Can you work these out from the model? Positions are in its coordinate system, mm. Face numbers are marked on the shaded views. A direction names the side the tool comes from. Give positions to 0.01 mm unless a question says otherwise; leave off trailing zeros. Write each loop counter-clockwise with the first axis right and the second up, starting at its lowest first coordinate (ties: lowest second). Pieces come first, ordered by that corner, then holes.
Autodesk Inventor part; units mm, degrees
ref_plane "Work Plane1" through (0, 190, 0) normal (0, 1, 0) x (-1, 0, 0)
ref_plane "Work Plane3" through (135, 0, 0) normal (1, 0, 0) x (0, 1, 0)
ref_plane "XY Plane" through (0, 0, 0) normal (0, 0, 1) x (1, 0, 0)
sketch "Sketch1" plane through (0, 0, 0) normal (0, 0, 1) x (1, 0, 0)
  line L0 (0, 0) -> (270, 0)
  line L1 (270, 0) -> (270, 380)
  line L2 (270, 380) -> (0, 380)
  line L3 (0, 380) -> (0, 0)
  dimension "d0" = 270
  dimension "d1" = 380
extrude "Extrusion1" add sketch "Sketch1" along normal blind 5
sketch "Sketch4" plane through (0, 0, 0) normal (-1, 0, 0) x (0, 0, 1)
  line L0 (0, 0) -> (0, 380)
  line L1 (-3.8919, 9.8795) -> (0, 9.8795)
  line L2 (0, 9.8795) -> (0, 5.6882)
  line L3 (0, 5.6882) -> (-3.8919, 5.6882)
  line L4 (-3.8919, 5.6882) -> (-3.8919, 9.8795)
  line L5 (5, 0) -> (5, 380)
  line L6 (5, 380) -> (87, 380)
  line L7 (87, 380) -> (87, 0)
  line L8 (87, 0) -> (5, 0)
  line L9 (5, 0) -> (5, 380)
  dimension "d4" = 82
  dimension "d5" = 380
extrude "Extrusion2" add sketch "Sketch4" against normal blind 5 contours L5 L6 L7 L8
sketch "Sketch7" plane through (0, 0, 0) normal (-1, 0, 0) x (0, 0, 1)
  line L0 (0, 380) -> (87, 380)
  line L1 (87, 380) -> (92, 380)
  line L2 (92, 380) -> (92, 0)
  line L3 (92, 0) -> (87, 0)
  line L4 (87, 0) -> (87, 380)
  point P0 (0, 0)
  dimension "d8" = 5
  dimension "d9" = 380
extrude "Extrusion3" add sketch "Sketch7" along normal blind 65 and the other way blind 5
sketch "Sketch8" plane through (0, 0, 0) normal (-1, 0, 0) x (0, 0, 1)
  line L0 (0, 380) -> (5, 380)
  line L1 (0, 380) -> (0, 390)
  line L2 (0, 390) -> (1.5922, 390)
  line L3 (5, 380) -> (92, 380)
  arc A0 (92, 380) -> (28.5, 443.5) centre (28.5, 380) ccw
  line L4 (28.5, 408.706) -> (28.5, 443.5)
  line L5 (57.206, 380) -> (92, 380)
  arc A1 (57.206, 380) -> (28.5, 408.706) centre (28.5, 380) ccw
  arc A2 (1.5922, 390) -> (0, 383.4325) centre (28.5, 380) ccw
  point P0 (0, 0)
  dimension "d14" = 10
extrude "Extrusion4" add sketch "Sketch8" along normal blind 65 and the other way blind 5 contours A1 L4 A0 L3
ref_plane "Work Plane1" through (0, 190, 0) normal (0, 1, 0) x (-1, 0, 0)
mirror "Mirror1" about plane through (0, 190, 0) normal (0, 1, 0) of "Extrusion4"
ref_plane "Work Plane3" through (135, 0, 0) normal (1, 0, 0) x (0, 1, 0)
mirror "Mirror2" about plane through (135, 0, 0) normal (1, 0, 0) of "Extrusion4", "Extrusion3", "Mirror1", "Extrusion2"
fillet "Fillet1" radius 2 3 edges at (5, -44.9013, 73.4013) (5, 424.9013, 73.4013) (5, 190, 92)
fillet "Fillet2" radius 2 3 edges at (265, 190, 92) (265, -44.9013, 73.4013) (265, 424.9013, 73.4013)
fillet "Fillet3" radius 2 1 edges at (5, 190, 5)
fillet "Fillet4" radius 2 1 edges at (265, 190, 5)
fillet "Fillet5" radius 2 1 edges at (0, 190, 0)
fillet "Fillet6" radius 2 1 edges at (270, 190, 0)
sketch "Sketch9" plane through (0, 0, 5) normal (0, 0, 1) x (1, 0, 0)
  line L0 (7, 0) -> (263, 0) construction
  line L1 (135, 0) -> (135, 150) construction
  circle A0 centre (135, 150) radius 12.5
  line L2 (135, 150) -> (258, 150) construction
  line L3 (135, 150) -> (12, 150) construction
  circle A1 centre (210, 150) radius 5
  circle A2 centre (60, 150) radius 5
  line L4 (5, 0) -> (5, 380)
  line L5 (265, 380) -> (265, 0)
  point P0 (0, 0)
  dimension "d27" = 150
  dimension "d28" = 25
  dimension "d31" = 10
  dimension "d32" = 10
  dimension "d33" = 55
  dimension "d34" = 55
extrude "Extrusion5" cut sketch "Sketch9" against normal through all
properties part number "body base" material "Steel, Alloy"
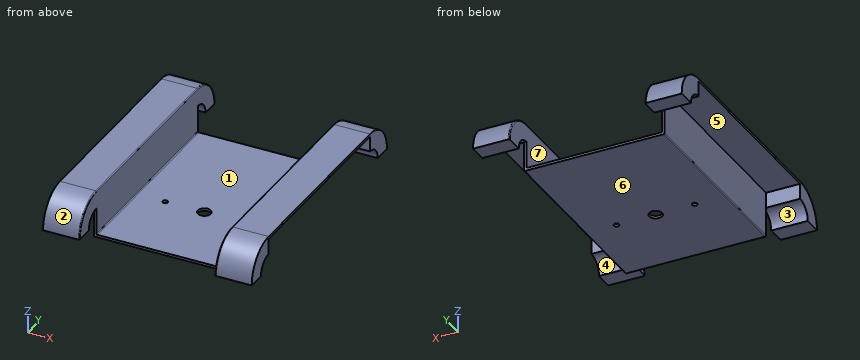
(1) If we mould it in two halves opening along Y, with no side actions, what happens to the marked faces 1, 2 and 3? For each: +Y half, -Y half, draft (parallel to the pull), parting line (faces both ways), or undercut.
Returned:
face 1: draft
face 2: -Y half
face 3: undercut
(2) Imagine slicing it at B-B, the plane y = 206.5. Write out the boundary of the cut face in (x, z).
Returned:
outline: (-65, 87) - (0, 87) - (0, 2) arc R2 ccw to (2, 0) - (268, 0) arc R2 ccw to (270, 2) - (270, 87) - (335, 87) - (335, 92) - (267, 92) arc R2 ccw to (265, 90) - (265, 7) arc R2 cw to (263, 5) - (7, 5) arc R2 cw to (5, 7) - (5, 90) arc R2 ccw to (3, 92) - (-65, 92) - close
(3) Imagine slicing it at D-D, the plane x = 182. Write out the boundary of the cut face in (y, z), plus the area to 3 significant figures.
Returned:
outline: (0, 0) - (380, 0) - (380, 5) - (0, 5) - close
area: 1,900 mm2
(4) For the marked faces 4, 5, 6 and 7, which set-ups out of +Z, -Z, +X, -X, +Y, -Y let a thin tool reach every point of the face, with its end or its side?
Returned:
face 4: -Z, +X, -X
face 5: -Z, -X
face 6: -Z, +X, -X, +Y, -Y
face 7: +Z, +Y, -Y
(5) Imagine slicing it at A-A, the plane x = 135. Write out the boundary of the cut face in (y, z).
Returned:
outline: (0, 0) - (137.5, 0) - (137.5, 5) - (0, 5) - close; (162.5, 0) - (380, 0) - (380, 5) - (162.5, 5) - close
(6) If I drill on L1, parallel to X at y = 22, z = 36; L2, parallel to Y at x = 60, z = 3; L3, parallel to Y at x = 135, z = 1.65, over which ranges is the centre line in solid material (lowest first)?
Returned:
L1: x = 0 to 5, 265 to 270
L2: y = 0 to 145, 155 to 380
L3: y = 0 to 137.5, 162.5 to 380
(7) Will these pins go through, and if not, where does the flat tip stop? P1, Ø24, axis at x = 295, z = 67.5, coming from the +Y side; P2, Ø4, axis at y = 168, z = 17, coming from the +X side; P3, Ø15, axis at x = -20.5, z = 71, coming from the +Y side; P4, Ø8, axis at x = 60, y = 150, coming from the -Z side.
Returned:
P1: stops at y = 437.47
P2: stops at x = 270
P3: stops at y = 432.98
P4: passes through
(8) Imagine slicing it at C-C, the plane x = -11. Write out the boundary of the cut face in (y, z), plus the area to 3 significant figures.
Returned:
outline: (-63.5, 28.5) - (-28.71, 28.5) arc R28.71 cw to (0, 57.21) - (0, 87) - (380, 87) - (380, 57.21) arc R28.71 cw to (408.71, 28.5) - (443.5, 28.5) arc R63.5 ccw to (380, 92) - (0, 92) arc R63.5 ccw to start
area: 6,940 mm2
